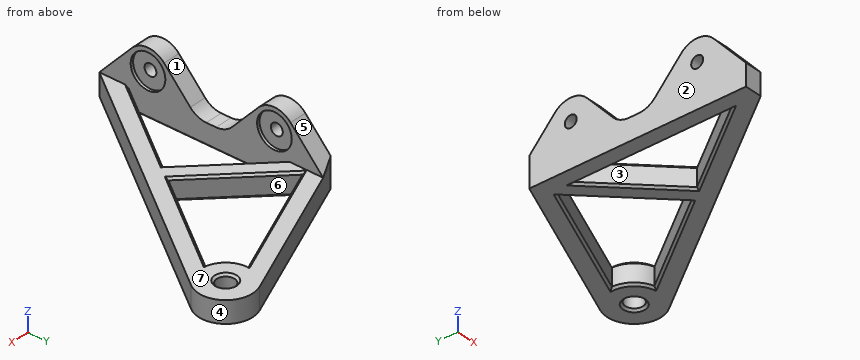
```python
from build123d import *

# Parameters (mm, degrees)
SKETCH_R        = 4.1
PAD_DEPTH       = 10
POCKET_DEPTH    = 10
PAD001_DEPTH    = 20
POCKET001_DEPTH = 10
CHAMFER_SIZE    = 1
CHAMFER001_SIZE = 1
SKETCH004_R     = 2.75
POCKET002_DEPTH = 8.001
SKETCH005_R     = 8
POCKET003_DEPTH = 1.3
FILLET_R        = 10


with BuildPart() as part:
    # Sketch → Pad (new body)
    with BuildSketch(Plane.XY):
        with BuildLine():
            Line((0, 0), (0, 100))
            Line((0, 100), (75.165103, 131.527089))
            ThreePointArc((90.101368, 112.637096), (89.805197, 127.752942), (75.165103, 131.527089))
            Line((90.101368, 112.637096), (8, 0))
            Line((8, 0), (0, 0))
        make_face()
        with Locations((80, 120)):
            Circle(SKETCH_R, mode=Mode.SUBTRACT)
    extrude(amount=PAD_DEPTH)

    # Sketch001 (on DatumPlane) → Pocket (cut)
    with BuildSketch(Plane.XY.offset(10)):
        Polygon((8, 13.581597), (8, 86.343146), (38.676131, 55.667014), align=None)
        with BuildLine():
            ThreePointArc((67.505213, 119.639023), (70.194803, 112.247058), (76.767254, 107.92526))
            Line((76.767254, 107.92526), (43.445969, 62.210885))
            Line((10.097006, 95.559849), (43.445969, 62.210885))
            Line((67.505213, 119.639023), (10.097006, 95.559849))
        make_face()
    extrude(amount=-POCKET_DEPTH, mode=Mode.SUBTRACT)

    # Sketch003 (on DatumPlane) → Pad001 (join)
    with BuildSketch(Plane.XY.offset(10)):
        Polygon((0, 100), (0, 0), (8, 0), (8, 103.355503), align=None)
    extrude(amount=PAD001_DEPTH)

    # Sketch002 (on DatumPlane) → Pocket001 (cut)
    with BuildSketch(Plane.YZ.offset(8)):
        with BuildLine():
            Line((0, 10), (15.077323, 26.70103))
            ThreePointArc((29.922685, 26.70103), (22.500004, 30), (15.077323, 26.70103))
            Line((29.922685, 26.70103), (45, 10))
            Line((45, 10), (58.355503, 10))
            Line((73.432722, 26.701024), (58.355503, 10))
            ThreePointArc((88.278096, 26.701024), (80.855409, 30), (73.432722, 26.701024))
            Line((103.355503, 10), (88.278096, 26.701024))
            Line((103.355503, 10), (128.355503, 10))
            Line((128.355503, 50), (128.355503, 10))
            Line((-25, 50), (128.355503, 50))
            Line((-25, 10), (-25, 50))
            Line((0, 10), (-25, 10))
        make_face()
    extrude(amount=-POCKET001_DEPTH, mode=Mode.SUBTRACT)

    # Chamfer
    chamfer_edges = [part.edges().sort_by_distance(p)[0] for p in [
        (75.9, 120, 10),
        (75.9, 120, 0),
    ]]
    chamfer(chamfer_edges, length=CHAMFER_SIZE)

    # Chamfer001
    chamfer001_edges = [part.edges().sort_by_distance(p)[0] for p in [
        (38.801109, 107.599436, 10),
        (70.194803, 112.247058, 10),
        (60.106612, 85.068072, 10),
        (26.771487, 78.885367, 10),
        (23.338066, 71.00508, 10),
        (23.338066, 34.624306, 10),
        (70.194803, 112.247058, 0),
        (60.106612, 85.068072, 0),
        (26.771487, 78.885367, 0),
        (38.801109, 107.599436, 0),
        (23.338066, 34.624306, 0),
        (8, 49.962371, 0),
        (23.338066, 71.00508, 0),
    ]]
    chamfer(chamfer001_edges, length=CHAMFER001_SIZE)

    # Sketch004 (on DatumPlane) → Pocket002 (cut, through all)
    with BuildSketch(Plane.YZ.offset(8)):
        with Locations((22.500004, 20)):
            Circle(SKETCH004_R)
        with Locations((80.855409, 20)):
            Circle(SKETCH004_R)
    extrude(amount=-POCKET002_DEPTH, mode=Mode.SUBTRACT)

    # Sketch005 (on DatumPlane) → Pocket003 (cut)
    with BuildSketch(Plane.YZ.offset(8)):
        with Locations((22.500004, 20)):
            Circle(SKETCH005_R)
        with Locations((80.855409, 20)):
            Circle(SKETCH005_R)
    extrude(amount=-POCKET003_DEPTH, mode=Mode.SUBTRACT)

    # Fillet
    fillet_edges = [part.edges().sort_by_distance(p)[0] for p in [
        (4, 58.355503, 10),
        (4, 45, 10),
    ]]
    fillet(fillet_edges, radius=FILLET_R)


solid = part.part
```
Build history of the part. All positions in model axes, mm. Face numbers are marked on the shaded views. A direction names the side the tool comes from. Round coordinates to 2 decimals unless told otherwise and drop trailing zeros. Write each loop counter-clockwise with the first axis right and the second up, starting at its lowest first coordinate (ties: lowest second). Pieces come first, ordered by that corner, then holes. Notation, with made-up numbers: (-10.75, -19) - (-2.75, -19) arc R8 ccw to (-2.75, -14) - close; hole circle Ø5 at (-9.5, 73.25). An arc over 180 degrees is marked (long way). Write each question's results on one line, items separated by ' | '. Start each with the question number.
Item 1: Which spindle directions (+Z, -Z, +X, -X, +Y, -Y) get a long thin tool onto all of the face, cutting with end or side? Do the marked faces 1, 2 and 3. Say none if no direction does.
Item 2: Drop flat-ended pins along their axis: P1, Ø8, axis at y = 84.5, z = 16.5, coming from the +X side; P2, Ø5, axis at x = 58.5, y = 75.5, coming from the +Z side; P3, Ø2, axis at x = 17, z = 6.5, coming from the +Y side. Give the stop position or say it passes through.
Item 3: Saw through at B-B (y = 94). Write the cut outline in (x, z), and give its area (3 significant figures).
Item 4: Saw through at A-A (z = 7.5). Write the cut outline in (x, y).
Item 5: Saw through at D-D (y = 70). Write the cut outline in (x, z), and give its area (3 significant figures).
Item 6: Mould opens along Y. For the marked faces 4, 5, 6 and 7 say: pulls with the +Y half, pulls with the -Y half, needs draft (parallel to the pull), parting line crosses it, or undercut.
Item 7: Wall check: L1, parallel to X at y = 68, z = 4; L2, parallel to Y at x = 29, z = 3.5; L3, parallel to X at y = 34, z = 12. Give the ranges that are in metal, low to high. Write a range as [from, to].
Item 8: Saw through at C-C (z = 20). Write the cut outline in (x, y), and give its area (3 significant figures).
Results are:
1) face 1: +Z, +X, -X | face 2: +Z, -Z, -X, +Y, -Y | face 3: +Z, -Z
2) P1: stops at x = 8 | P2: stops at z = 10 | P3: stops at y = 107.55
3) outline: (0, 0) - (10.24, 0) - (11.66, 1) - (11.66, 9) - (10.24, 10) - (8, 10) - (8, 20.36) - (0, 20.36) - close; (66.62, 1) - (67.85, 0) - (76.52, 0) - (76.52, 10) - (67.85, 10) - (66.62, 9) - close | area: 296 mm²
4) outline: (0, 0) - (8, 0) - (90.1, 112.64) arc R12.5 ccw to (75.17, 131.53) - (0, 100) - close; hole (8, 13.58) - (38.68, 55.67) - (8, 86.34) - close; hole (10.1, 95.56) - (43.45, 62.21) - (76.77, 107.93) arc R12.5 cw to (67.51, 119.64) - close; hole circle Ø8.2 at (80, 120)
5) outline: (0, 0) - (7, 0) - (8, 1) - (8, 22.9) - (0, 22.9) - close; (24.34, 1) - (25.76, 0) - (34.24, 0) - (35.66, 1) - (35.66, 9) - (34.24, 10) - (25.76, 10) - (24.34, 9) - close; (49.12, 1) - (50.36, 0) - (59.02, 0) - (59.02, 10) - (50.36, 10) - (49.12, 9) - close | area: 391 mm²
6) face 4: parting line crosses it | face 5: pulls with the +Y half | face 6: undercut | face 7: needs draft
7) L1: x = [0, 8], [26.34, 37.66], [47.67, 57.57] | L2: y = [28.81, 42.39], [65.34, 76.66], [103.49, 112.16] | L3: x = [0, 8]
8) outline: (0, 9.03) - (8, 9.03) - (8, 14.5) - (6.7, 14.5) - (6.7, 19.75) - (0, 19.75) - close; (0, 25.25) - (6.7, 25.25) - (6.7, 30.5) - (8, 30.5) - (8, 35.97) - (0, 35.97) - close; (0, 67.38) - (8, 67.38) - (8, 72.86) - (6.7, 72.86) - (6.7, 78.11) - (0, 78.11) - close; (0, 83.61) - (6.7, 83.61) - (6.7, 88.86) - (8, 88.86) - (8, 94.33) - (0, 94.33) - close | area: 316 mm²
